Input: part model. Units: mm. Frame: model coordinates. Give positions to 0.01 mm unless a question says otherwise; leave off trailing zeros. Loops run counter-clockwise (first coordinate to the right, second up) from the corner with the lowest first, then second, coordinate; pieces in that order, holes last. Notation, with made-up numbers: M 25.5,10 L 29.5,10 A23 cw 29.5,39 Z; hole C 55,66.25 d7. An arc over 180 degrees is marked long. One line per item, written item: value. Start each with the question number.
(1) Ray query, line 1 along Y through (x, z) = (0, 44.5); line 2 along X through (y, z) = (0, 26); line 3 along X through (y, z) = (-0.25, 71.5). Return the intervals inside material, ascending. Write a range as from..to.
(2) Pin query (flat end, axial travel): P1, Ø2, axis at x = -3, z = 40, coming from the +Y side. Return the tip coordinate at first contact, or that it passes through.
(3) Section A-A on z = 47. Output: boundary loops of the cut face in (x, y).
Autodesk Inventor part; units mm, degrees
ref_plane "YZ Plane" through (0, 0, 0) normal (1, 0, 0) x (0, 1, 0)
ref_plane "XZ Plane" through (0, 0, 0) normal (0, 1, 0) x (-1, 0, 0)
ref_plane "XY Plane" through (0, 0, 0) normal (0, 0, 1) x (1, 0, 0)
sketch "Sketch1" plane through (0, 0, 0) normal (0, 0, 1) x (1, 0, 0)
  line L0 (-6.35, -3.6662) -> (-6.35, 3.6662)
  line L1 (-6.35, 3.6662) -> (0, 7.3323)
  line L2 (0, 7.3323) -> (6.35, 3.6662)
  line L3 (6.35, 3.6662) -> (6.35, -3.6662)
  line L4 (6.35, -3.6662) -> (0, -7.3323)
  line L5 (0, -7.3323) -> (-6.35, -3.6662)
  point P0 (0, 0)
  point P1 (0, 0)
  dimension "Size" = 12.7
extrude "Extrusion1" add sketch "Sketch1" along normal mid plane 157.1625
sketch "Sketch3" plane through (0, 0, 78.5812) normal (0, 0, 1) x (1, 0, 0)
  line L0 (-6.35, 3.6662) -> (0, 7.3323) construction
  line L1 (0, 7.3323) -> (6.35, 3.6662) construction
  line L2 (6.35, 3.6662) -> (6.35, -3.6662) construction
  line L3 (6.35, -3.6662) -> (0, -7.3323) construction
  line L4 (0, -7.3323) -> (-6.35, -3.6662) construction
  line L5 (-6.35, -3.6662) -> (-6.35, 3.6662) construction
  point P0 (0, 0)
hole "Hole1" at (0, 0, 78.5812) direction (0, 0, -1) diameter 5.1054 end through all
sketch "Sketch4" plane through (0, 0, 78.5812) normal (0, 0, 1) x (1, 0, 0)
  circle A0 centre (0, 0) radius 2.5527 construction
  line L0 (-6.35, 3.6662) -> (0, 7.3323) construction
  line L1 (0, 7.3323) -> (6.35, 3.6662) construction
  line L2 (6.35, 3.6662) -> (6.35, -3.6662) construction
  line L3 (6.35, -3.6662) -> (0, -7.3323) construction
  line L4 (0, -7.3323) -> (-6.35, -3.6662) construction
  line L5 (-6.35, -3.6662) -> (-6.35, 3.6662) construction
  circle A1 centre (0, 0) radius 6.8771
  circle A2 centre (0, 0) radius 8.89
  dimension "thunder" = 13.7541
  dimension "d16" = 17.78
extrude "Extrusion3" cut sketch "Sketch4" against normal through all
sketch "Sketch5" plane through (0, 0, 78.5812) normal (0, 0, 1) x (1, 0, 0)
  circle A0 centre (0, 0) radius 6.35
  arc A1 (5.4616, -4.1791) -> (6.35, -2.6403) centre (0, 0) ccw
  line L0 (6.35, -2.6403) -> (6.35, 2.6403)
  arc A2 (6.35, 2.6403) -> (5.4616, 4.1791) centre (0, 0) ccw
  line L1 (5.4616, 4.1791) -> (0.8884, 6.8194)
  arc A3 (0.8884, 6.8194) -> (-0.8884, 6.8194) centre (0, 0) ccw
  line L2 (-0.8884, 6.8194) -> (-5.4616, 4.1791)
  arc A4 (-5.4616, 4.1791) -> (-6.35, 2.6403) centre (0, 0) ccw
  line L3 (-6.35, 2.6403) -> (-6.35, -2.6403)
  arc A5 (-6.35, -2.6403) -> (-5.4616, -4.1791) centre (0, 0) ccw
  line L4 (-5.4616, -4.1791) -> (-0.8884, -6.8194)
  arc A6 (-0.8884, -6.8194) -> (0.8884, -6.8194) centre (0, 0) ccw
  line L5 (0.8884, -6.8194) -> (5.4616, -4.1791)
  circle A7 centre (0, 0) radius 2.5527 construction
  point P0 (3.175, -5.4993)
  point P1 (-3.175, -5.4993)
  point P2 (-6.35, 0)
  point P3 (-3.175, 5.4993)
  point P4 (3.175, 5.4993)
  point P5 (6.35, 0)
  dimension "d19" = 12.7
extrude "Extrusion4" cut sketch "Sketch5" against normal blind 8.001 contours L0 A1 L5 A0 | A0 L1 A2 L0 | A0 L2 A3 L1 | L5 A6 L4 A0 | A0 L3 A4 L2 | L4 A5 L3 A0
equation "\"bearing\" = 25.4"
properties part number "GP5-009" material "Aluminum 6061"
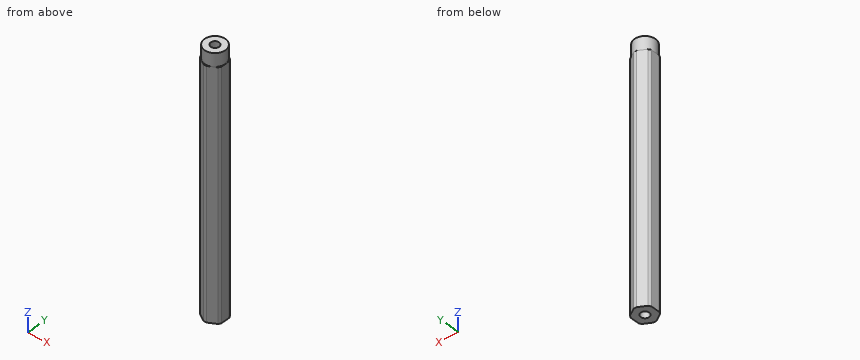
Output values:
1. line 1: y = -6.88..-2.55, 2.55..6.88
1. line 2: x = -6.35..-2.55, 2.55..6.35
1. line 3: x = -6.35..-2.54, 2.54..6.35
2. P1: stops at y = 6.18
3. outline: M -6.35,-2.64 A6.88 ccw -5.46,-4.18 L -0.89,-6.82 A6.88 ccw 0.89,-6.82 L 5.46,-4.18 A6.88 ccw 6.35,-2.64 L 6.35,2.64 A6.88 ccw 5.46,4.18 L 0.89,6.82 A6.88 ccw -0.89,6.82 L -5.46,4.18 A6.88 ccw -6.35,2.64 Z; hole C 0,0 d5.11
